Work out the finished part from the listing and answer in its coordinate system (mm). A direction names the side the tool comes from. Round coordinates to 2 decimals unless told otherwise and drop trailing zeros. Order: outer loops, then holes, each group sorted by start corner. A loop starts at its lowest first (then second) coordinate and runs counter-clockwise, first axis right, second up. Notation, with made-up numbers: M -14,-15.75 L -4,-15.75 A17 ccw -4,-0.75 Z; hole C -23.75,-36.75 d2. An arc over 180 degrees is marked long. Answer as a JSON object with one key per item and string values. Group by question number.
from build123d import *

# Parameters (mm, degrees)
F0_R     = 19
F0_R_2   = 2.25
F1_DEPTH = 6
F2_R     = 3


with BuildPart() as f1:
    # F0 (on Top) → F1 (new body)
    with BuildSketch(Plane.XY):
        with Locations((-65, 34.5)):
            Circle(F0_R)
        with Locations((-65, 18.5)):
            Circle(F0_R_2, mode=Mode.SUBTRACT)
        with Locations((-77, 34.5)):
            Circle(F0_R_2, mode=Mode.SUBTRACT)
        with BuildLine():
            ThreePointArc((-68.461639, 20.965675), (-74.671252, 24.418939), (-78.3791, 30.479977))
            ThreePointArc((-78.3791, 30.479977), (-72.75, 34.5), (-78.3791, 38.520023))
            ThreePointArc((-78.3791, 38.520023), (-74.671252, 44.581061), (-68.461639, 48.034325))
            ThreePointArc((-68.461639, 48.034325), (-65, 46.25), (-61.538361, 48.034325))
            ThreePointArc((-61.538361, 48.034325), (-55.328748, 44.581061), (-51.6209, 38.520023))
            ThreePointArc((-51.6209, 38.520023), (-57.25, 34.5), (-51.6209, 30.479977))
            ThreePointArc((-51.6209, 30.479977), (-55.328748, 24.418939), (-61.538361, 20.965675))
            ThreePointArc((-61.538361, 20.965675), (-65, 22.75), (-68.461639, 20.965675))
        make_face(mode=Mode.SUBTRACT)
        with Locations((-53, 34.5)):
            Circle(F0_R_2, mode=Mode.SUBTRACT)
        with Locations((-65, 50.5)):
            Circle(F0_R_2, mode=Mode.SUBTRACT)
    extrude(amount=-F1_DEPTH)

    # F2
    f2_edges = [f1.edges().sort_by_distance(p)[0] for p in [
        (-61.538361, 20.965675, -3),
        (-68.461639, 20.965675, -3),
        (-78.3791, 30.479977, -3),
        (-78.3791, 38.520023, -3),
        (-51.6209, 30.479977, -3),
        (-68.461639, 48.034325, -3),
        (-61.538361, 48.034325, -3),
        (-51.6209, 38.520023, -3),
    ]]
    fillet(f2_edges, radius=F2_R)


solid = f1.part
Item 1: Find section A-A (y = 35). Give the vertices of the cut face in (x, z).
Item 2: The mould has two halves that part along Y. Classify faces 1 (the flat face through (-57, 35, -6)), 2 (the cylindrical face through (-57.25, 34.57, -2.96)), 3 (the cylindrical face through (-80.08, 22.94, -2.96)): +Y half, -Y half, draft (parallel to the pull), parting line (faces both ways), or undercut.
Item 3: Each of these flat-tipped pins is pushed along its axis until it touches: pin 1 (1 mm diameter, centred on x = -65, z = -2.5, fed in from -Y); pin 2 (1.5 mm diameter, centred on y = 20, z = -4.5, fed in from +X); pin 3 (2 mm diameter, centred on y = 47.5, z = -5.5, fed in from +X). Where does it stop, or does it pass through?
Item 4: Find section C-C (z = -5). Give the number of separate pieces and of enclosed holes in the cut face, and give its area (3 significant figures).
Item 5: Consider L1, parallel to Y at x = -65, z = -1.65; L2, parallel to X at y = 28, z = -3.5; L3, parallel to Y at x = -71.5, z = -2. Determine where each line is inside the solid, lowest interval first.
Item 6: Find section D-D (y = 24). Give the vertices of the cut face in (x, z).
Item 7: A tool of negligible diameter and unlimited length cuts with its end or side. For faces 4 (the cylindrical face through (-65.04, 46.25, -2.96)), 5 (the flat face through (-57, 35, 0)), from which of +Z, -Z, +X, -X, +Y, -Y can it reach the whole face along a straight path? Write none if from no direction.
Item 8: Find section B-B (x = -71.5). Give the vertices of the cut face in (y, z).
Responses:
{
 "1": {"outline": "M -83.99,-6 L -79.19,-6 L -79.19,0 L -83.99,0 Z; M -74.81,-6 L -72.78,-6 L -72.78,0 L -74.81,0 Z; M -57.22,-6 L -55.19,-6 L -55.19,0 L -57.22,0 Z; M -50.81,-6 L -46.01,-6 L -46.01,0 L -50.81,0 Z"},
 "2": {"face 1": "draft", "face 2": "undercut", "face 3": "parting line"},
 "3": {"pin 1": "stops at y = 15.5", "pin 2": "stops at x = -51.89", "pin 3": "stops at x = -50.27"},
 "4": {"separate pieces": "1", "enclosed holes": "5", "area": "581 mm^2"},
 "5": {"L1": "y = 15.5 to 16.25, 20.75 to 22.75, 46.25 to 48.25, 52.75 to 53.5", "L2": "x = -82.85 to -76.82, -53.18 to -47.15", "L3": "y = 16.65 to 22.13, 46.87 to 52.35"},
 "6": {"outline": "M -80.84,-6 L -74.21,-6 L -74.21,0 L -80.84,0 Z; M -55.79,-6 L -49.16,-6 L -49.16,0 L -55.79,0 Z"},
 "7": {"face 4": "+Z, -Z", "face 5": "+Z, +X, -X, +Y, -Y"},
 "8": {"outline": "M 16.65,-6 L 22.13,-6 L 22.13,0 L 16.65,0 Z; M 46.87,-6 L 52.35,-6 L 52.35,0 L 46.87,0 Z"}
}
